For this review, take the finished solid that the model builds, in its own axes (mm). Face numbers are marked on the shaded views. A direction names the side the tool comes from. Round coordinates to 2 decimals unless told otherwise and drop trailing zeros. Write each loop counter-clockwise with the first axis right and the second up, starting at its lowest first coordinate (ties: lowest second). Pieces come first, ordered by that corner, then holes. Notation, with made-up numbers: (54.25, -22.5) - (112.25, -22.5) arc R18 cw to (112.25, 0.5) - close; hole circle Ø8 at (-18.5, 88.5). An arc over 180 degrees is marked (long way). Answer in a Markdown table with one row per item. Add a question column.
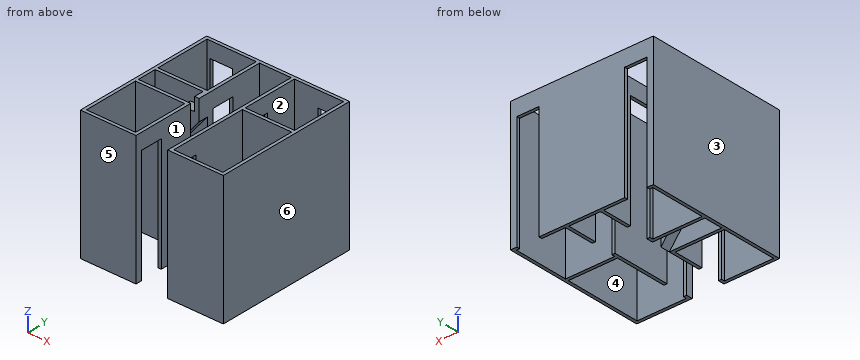
from build123d import *

# Parameters (mm, degrees)
F0_W          = 393.7
F0_H          = 25.4
F0_W_2        = 25.4
F0_H_2        = 241.3
F0_H_3        = 444.5
F0_H_4        = 152.4
F0_H_5        = 12.7
F1_DEPTH      = 1016
F1_DEPTH_BACK = 25.4
F0_W_3        = 190.5
F0_W_4        = 254
F0_H_6        = 419.1
F0_H_7        = 622.3
F2_W          = 177.8
F2_H          = 25.4
F2_W_2        = 25.4
F2_H_2        = 177.8
F3_DEPTH      = 127
F5_W          = 152.4
F5_H          = 127
F6_DEPTH      = 76.2
F10_W         = 14.2358661652
F10_H         = 119.38
F11_DEPTH     = 76.2
F12_DEPTH     = 76.2


with BuildPart() as f1:
    # F0 (on Top) → F1 (new body, two sides)
    with BuildSketch(Plane.XY) as f1_sk:
        with Locations((-349.25, -88.9)):
            Rectangle(F0_W, F0_H)
        with Locations((-139.7, -88.9)):
            Rectangle(F0_W_2, F0_H)
        with Locations((-139.7, -222.25)):
            Rectangle(F0_W_2, F0_H_2)
        with Locations((-558.8, -323.85)):
            Rectangle(F0_W_2, F0_H_3)
        with Locations((-558.8, -88.9)):
            Rectangle(F0_W_2, F0_H)
        with Locations((-558.8, 0)):
            Rectangle(F0_W_2, F0_H_4)
        with Locations((-558.8, 82.55)):
            Rectangle(F0_W_2, F0_H_5)
        with Locations((-558.8, 95.25)):
            Rectangle(F0_W_2, F0_H_5)
        with Locations((-558.8, 323.85)):
            Rectangle(F0_W_2, F0_H_3)
        with Locations((-558.8, 558.8)):
            Rectangle(F0_W_2, F0_H)
        with Locations((-533.4, 558.8)):
            Rectangle(F0_W_2, F0_H)
        Polygon((-152.4, 101.6), (-127, 101.6), (-127, 103.0518114567), (-127, 127), (-152.4, 127), align=None)
        Polygon((-152.4, 88.9), (-152.4, 76.2), (-127, 76.2), (-127, 101.6), (-152.4, 101.6), align=None)
        with Locations((-349.25, 95.25)):
            Rectangle(F0_W, F0_H_5)
        with Locations((-349.25, 82.55)):
            Rectangle(F0_W, F0_H_5)
        with Locations((-139.7, -533.4)):
            Rectangle(F0_W_2, F0_H)
        with Locations((-349.25, -558.8)):
            Rectangle(F0_W, F0_H)
        with Locations((-558.8, -558.8)):
            Rectangle(F0_W_2, F0_H)
        with Locations((-139.7, -558.8)):
            Rectangle(F0_W_2, F0_H)
    extrude(amount=F1_DEPTH)
    extrude(f1_sk.sketch, amount=-F1_DEPTH_BACK)



with BuildPart() as f1b:
    # F0 (on Top) → F1, piece 2 (new body, two sides)
    with BuildSketch(Plane.XY) as f1_2_sk:
        with Locations((-247.65, 558.8)):
            Rectangle(F0_W_3, F0_H)
        with Locations((-139.7, 558.8)):
            Rectangle(F0_W_2, F0_H)
        with Locations((-139.7, 425.45)):
            Rectangle(F0_W_2, F0_H_2)
        with Locations((247.65, 558.8)):
            Rectangle(F0_W_3, F0_H)
        with Locations((139.7, 558.8)):
            Rectangle(F0_W_2, F0_H)
        with Locations((139.7, 425.45)):
            Rectangle(F0_W_2, F0_H_2)
        with Locations((0, 558.8)):
            Rectangle(F0_W_4, F0_H)
    extrude(amount=F1_DEPTH)
    extrude(f1_2_sk.sketch, amount=-F1_DEPTH_BACK)


with BuildPart() as f1c:
    # F0 (on Top) → F1, piece 3 (new body, two sides)
    with BuildSketch(Plane.XY) as f1_3_sk:
        with Locations((349.25, 82.55)):
            Rectangle(F0_W, F0_H_5)
        Polygon((152.4, 88.9), (546.1, 88.9), (546.1, 101.6), (152.4, 101.6), (152.4, 101.5882790089), align=None)
        Polygon((127, 101.6), (127, 88.9), (152.4, 88.9), (152.4, 101.5882790089), (152.4, 101.6), align=None)
        with Locations((139.7, 114.3)):
            Rectangle(F0_W_2, F0_H)
        with Locations((139.7, 82.55)):
            Rectangle(F0_W_2, F0_H_5)
        with Locations((139.7, -133.35)):
            Rectangle(F0_W_2, F0_H_6)
        with Locations((139.7, -533.4)):
            Rectangle(F0_W_2, F0_H)
        with Locations((139.7, -558.8)):
            Rectangle(F0_W_2, F0_H)
        with Locations((349.25, -558.8)):
            Rectangle(F0_W, F0_H)
        with Locations((558.8, -234.95)):
            Rectangle(F0_W_2, F0_H_7)
        with Locations((558.8, -558.8)):
            Rectangle(F0_W_2, F0_H)
        with Locations((558.8, 95.25)):
            Rectangle(F0_W_2, F0_H_5)
        with Locations((558.8, 82.55)):
            Rectangle(F0_W_2, F0_H_5)
        with Locations((558.8, 323.85)):
            Rectangle(F0_W_2, F0_H_3)
        with Locations((558.8, 558.8)):
            Rectangle(F0_W_2, F0_H)
        with Locations((533.4, 558.8)):
            Rectangle(F0_W_2, F0_H)
    extrude(amount=F1_DEPTH)
    extrude(f1_3_sk.sketch, amount=-F1_DEPTH_BACK)


with BuildPart() as f1_1:
    add(f1.part)

    add(f1b.part)  # F3 merges F1b

    add(f1c.part)  # F3 merges F1c
    # F2 (on face) → F3 (join)
    with BuildSketch(Plane.XY.offset(1016)):
        with Locations((-431.8, 558.8)):
            Rectangle(F2_W, F2_H)
        with Locations((-139.7, -431.8)):
            Rectangle(F2_W_2, F2_H_2)
        with Locations((139.7, -431.8)):
            Rectangle(F2_W_2, F2_H_2)
        with Locations((431.8, 558.8)):
            Rectangle(F2_W, F2_H)
        with Locations((139.7, 215.9)):
            Rectangle(F2_W_2, F2_H_2)
        with Locations((-139.7, 215.9)):
            Rectangle(F2_W_2, F2_H_2)
    extrude(amount=-F3_DEPTH)

    # F4: union 

    # F5 (on face) → F6 (join)
    with BuildSketch(Plane.YZ.offset(-546.1)):
        with Locations((0, 495.3)):
            Rectangle(F5_W, F5_H)
    extrude(amount=F6_DEPTH)

    # F10 (on offset) → F11 (join, through all)
    with BuildSketch(Plane.XZ):
        Polygon((-469.9, 678.18), (-469.9, 558.8), (-393.7, 558.8), (-393.7, 525.1186495463), (-127, 851.7339229584), (-127, 1016), (-162.56, 1016), (-162.56, 909.32), (-264.16, 909.32), (-264.16, 795.02), (-365.76, 795.02), (-365.76, 678.18), align=None)
        with Locations((-477.0179330826, 618.49)):
            Rectangle(F10_W, F10_H)
        Polygon((-393.7, 558.8), (-469.9, 558.8), (-469.9, 431.8), (-393.7, 525.1186495463), align=None)
    extrude(amount=-F11_DEPTH)

    # F10 (on offset) → F12 (join, through all)
    with BuildSketch(Plane.XZ):
        Polygon((-393.7, 525.1186495463), (-469.9, 431.8), (-469.9, 413.5754568294), (-127, -25.4), (-127, 5.08), (-127, 106.68), (-203.2, 106.68), (-203.2, 243.84), (-317.5, 243.84), (-317.5, 378.46), (-393.7, 378.46), (-393.7, 431.8), align=None)
        Polygon((-393.7, 558.8), (-469.9, 558.8), (-469.9, 431.8), (-393.7, 525.1186495463), align=None)
    extrude(amount=F12_DEPTH)


solid = f1_1.part
Q1. Tool access review of the marked faces 1, 2 and 3: name each direction out of +Z, -Z, +X, -X, +Y, -Y from which nothing blocks a thin tool from reaching the whole face with its end or side.
Q2. Add section C-C on y = 437. State the section outline as (x, z) points, then the cut area to 3 significant figures.
Q3. Draft analysis for pull direction X (two halves, no side actions). For the marked faces 4, 5 and 6, state which applies: released by +X, released by -X, zero draft, split by the parting line, or undercut.
Q4. To check wall thickness, follow probe 1 along X at (y, z) = (392, 622); probe 2 along Y at (x, z) = (276.5, 363.5); probe 3 along Y at (x, z) = (-159.5, 475.5). State the ranges of each line that lie inside material, in increasing order.
Q5. Insertion check: pin 1 Ø10 at (x, z) = (-432, 861.5) entering from +Y; pin 2 Ø12 at (x, y) = (-175.5, 47) entering from -Z; pin 3 Ø23 at (x, y) = (-202, 33) entering from +Z; pin 4 Ø6 at (x, y) = (123.5, -257.5) entering from +Z. Each pin has a flat end and moves straight along its axis. Give the tip position at first contact, or say it passes through.
Q6. Add section A-A on y = -499. State the section outline as (x, z) points.
Q7. Add section D-D on x = 459. State the section outline as (y, z) points.
Q8. Add section B-B on x = 285.5. State the section outline as (y, z) points.
Answer sheet:
| question | item | result |
|---|---|---|
| 1 | face 1 | +Z, -Z, -Y |
| 1 | face 2 | +Z, -Z |
| 1 | face 3 | +Z, -Z, -X, +Y, -Y |
| 2 | outline | (-571.5, -25.4) - (-546.1, -25.4) - (-546.1, 1016) - (-571.5, 1016) - close; (-152.4, -25.4) - (-127, -25.4) - (-127, 1016) - (-152.4, 1016) - close; (127, -25.4) - (152.4, -25.4) - (152.4, 1016) - (127, 1016) - close; (546.1, -25.4) - (571.5, -25.4) - (571.5, 1016) - (546.1, 1016) - close |
| 2 | area | 106,000 mm² |
| 3 | face 4 | undercut |
| 3 | face 5 | zero draft |
| 3 | face 6 | released by +X |
| 4 | probe 1 | x = -571.5 to -546.1, -152.4 to -127, 127 to 152.4, 546.1 to 571.5 |
| 4 | probe 2 | y = -571.5 to -546.1, 76.2 to 101.6, 546.1 to 571.5 |
| 4 | probe 3 | y = -571.5 to -546.1, -101.6 to -76.2, 76.2 to 101.6, 546.1 to 571.5 |
| 5 | pin 1 | stops at y = 101.6 |
| 5 | pin 2 | stops at z = 784.99 |
| 5 | pin 3 | stops at z = 909.32 |
| 5 | pin 4 | passes through |
| 6 | outline | (-571.5, -25.4) - (-546.1, -25.4) - (-546.1, 1016) - (-571.5, 1016) - close; (-152.4, 889) - (-127, 889) - (-127, 1016) - (-152.4, 1016) - close; (127, 889) - (152.4, 889) - (152.4, 1016) - (127, 1016) - close; (546.1, -25.4) - (571.5, -25.4) - (571.5, 1016) - (546.1, 1016) - close |
| 7 | outline | (-571.5, -25.4) - (-546.1, -25.4) - (-546.1, 1016) - (-571.5, 1016) - close; (76.2, -25.4) - (101.6, -25.4) - (101.6, 1016) - (76.2, 1016) - close; (546.1, 889) - (571.5, 889) - (571.5, 1016) - (546.1, 1016) - close |
| 8 | outline | (-571.5, -25.4) - (-546.1, -25.4) - (-546.1, 1016) - (-571.5, 1016) - close; (76.2, -25.4) - (101.6, -25.4) - (101.6, 1016) - (76.2, 1016) - close; (546.1, -25.4) - (571.5, -25.4) - (571.5, 1016) - (546.1, 1016) - close |
